Source: CAD feature listing. Evaluate the final solid. Frame: model axes, mm. Face numbers are marked on the shaded views. A direction names the side the tool comes from. Round coordinates to 2 decimals unless told otherwise and drop trailing zeros. Loops run counter-clockwise (first coordinate to the right, second up) from the corner with the lowest first, then second, coordinate; pieces in that order, holes last. Notation, with made-up numbers: (52.5, 4.5) - (109.5, 4.5) arc R16 ccw to (109.5, 21.5) - close; hole circle Ø7 at (60, 55). An arc over 180 degrees is marked (long way). Write item = value, one per line. Start each with the question number.
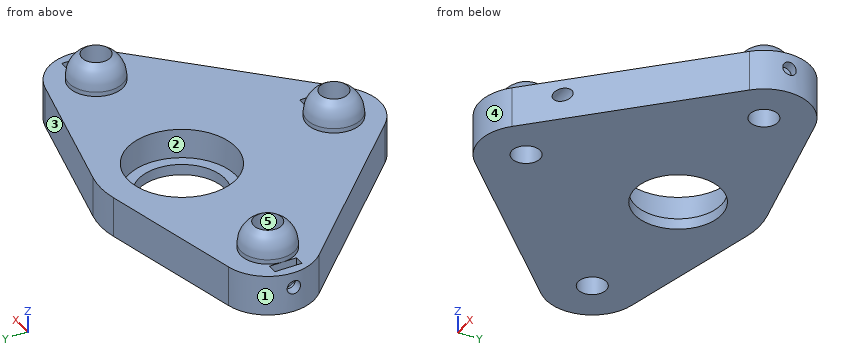
from build123d import *

# Parameters (mm, degrees)
F0_R        = 3.302
F0_R_2      = 12.7
F1_DEPTH    = 9.525
F0_R_3      = 10.16
F2_DEPTH    = 2.54
F5_DEPTH    = 8.636
F6_T1_DEPTH = 2.3368
F6_T3_DEPTH = 2.3368
F6_T5_DEPTH = 2.3368
F3_R        = 6.35
F3_R_2      = 3.302
F7_DEPTH    = 6.35
F11_R       = 1.5875
F12_DEPTH   = 6.35
F9_R        = 1.5875
F13_DEPTH   = 6.35
F10_R       = 1.5875
F14_DEPTH   = 8.382


# Not quite as in the source:
# - a fillet or chamfer that OpenCascade refuses, or shapes differently, is made with other operations: its cross-section is extruded or revolved along the edge and cut away or added
# - a feature names something its author has since deleted; it is built from what else it names


with BuildPart() as f1:
    # F0 (on Top) → F1 (new body)
    with BuildSketch(Plane.XY):
        with BuildLine():
            Line((38.3924752276, 46.5596586637), (4.3105120801, 54.476849111))
            ThreePointArc((4.3105120801, 54.476849111), (0, 54.970934), (-4.3105120801, 54.476849111))
            Line((-4.3105120801, 54.476849111), (-38.3924752276, 46.5596586637))
            ThreePointArc((-38.3924752276, 46.5596586637), (-46.4220600308, 38.9243049052), (-43.6441157783, 28.1978942818))
            Line((-43.6441157783, 28.1978942818), (-7.72300081, -7.7230397182))
            ThreePointArc((-7.72300081, -7.7230397182), (0, -10.922), (7.72300081, -7.7230397182))
            Line((7.72300081, -7.7230397182), (43.6441157783, 28.1978942818))
            ThreePointArc((43.6441157783, 28.1978942818), (46.4220600308, 38.9243049052), (38.3924752276, 46.5596586637))
        make_face()
        Circle(F0_R, mode=Mode.SUBTRACT)
        with Locations((-35.9211149683, 35.920934)):
            Circle(F0_R, mode=Mode.SUBTRACT)
        with Locations((0, 35.920934)):
            Circle(F0_R_2, mode=Mode.SUBTRACT)
        with Locations((35.9211149683, 35.920934)):
            Circle(F0_R, mode=Mode.SUBTRACT)
    extrude(amount=F1_DEPTH)

    # F0 (on Top) → F2 (join)
    with BuildSketch(Plane.XY):
        with Locations((0, 35.920934)):
            Circle(F0_R_2)
        with Locations((0, 35.920934)):
            Circle(F0_R_3, mode=Mode.SUBTRACT)
    extrude(amount=F2_DEPTH)

    # F4 (on face) → F5 (cut)
    with BuildSketch(Plane.XY.offset(9.525)):
        Polygon((-42.2711149683, 32.695134), (-42.2711149683, 35.920934), (-42.2711149683, 39.146734), (-44.6079149683, 39.146734), (-44.6079149683, 32.695134), align=None)
        Polygon((42.2711149683, 39.146734), (42.2711149683, 35.920934), (42.2711149683, 32.695134), (44.6079149683, 32.695134), (44.6079149683, 39.146734), align=None)
        Polygon((6.35, 3.2258), (6.35, 0), (6.35, -3.2258), (8.6868, -3.2258), (8.6868, 3.2258), align=None)
    extrude(amount=-F5_DEPTH, mode=Mode.SUBTRACT)

    # F6: chamfer of 3.175 x 5.499261314 on 6 edges, made by hand

    # F6_s2 → F6_t1 (join)
    with BuildSketch(Plane.YZ.offset(-44.6079149683)):
        Polygon((39.146734, 4.064), (33.647472686, 0.889), (39.146734, 0.889), align=None)
        Polygon((32.695134, 4.064), (38.194395314, 0.889), (32.695134, 0.889), align=None)
    extrude(amount=F6_T1_DEPTH)

    # F6_s4 → F6_t3 (join)
    with BuildSketch(Plane.YZ.offset(6.35)):
        Polygon((3.2258, 4.064), (-2.273461314, 0.889), (3.2258, 0.889), align=None)
        Polygon((-3.2258, 4.064), (2.273461314, 0.889), (-3.2258, 0.889), align=None)
    extrude(amount=F6_T3_DEPTH)

    # F6_s6 → F6_t5 (join)
    with BuildSketch(Plane.YZ.offset(42.2711149683)):
        Polygon((39.146734, 4.064), (33.647472686, 0.889), (39.146734, 0.889), align=None)
        Polygon((32.695134, 4.064), (38.194395314, 0.889), (32.695134, 0.889), align=None)
    extrude(amount=F6_T5_DEPTH)

    # F3 (on face) → F7 (join)
    with BuildSketch(Plane.XY.offset(9.525)):
        with Locations((-35.9211149683, 35.920934)):
            Circle(F3_R)
        with Locations((-35.9211149683, 35.920934)):
            Circle(F3_R_2, mode=Mode.SUBTRACT)
        Circle(F3_R)
        Circle(F3_R_2, mode=Mode.SUBTRACT)
        with Locations((35.9211149683, 35.920934)):
            Circle(F3_R)
        with Locations((35.9211149683, 35.920934)):
            Circle(F3_R_2, mode=Mode.SUBTRACT)
    extrude(amount=F7_DEPTH)

    # F8: fillet of radius 6.096 on 3 edges, made by hand

    # F8_s1 → F8_t2 (revolve, cut)
    with BuildSketch(Plane.XZ.offset(-35.920934)):
        with BuildLine():
            ThreePointArc((-29.5711149683, 10.5957091385), (-30.3878241069, 13.6437091385), (-32.6191149683, 15.875))
            Line((-32.6191149683, 15.875), (-29.5711149683, 15.875))
            Line((-29.5711149683, 15.875), (-29.5711149683, 10.5957091385))
        make_face()
    revolve(axis=Axis((-35.9211149683, 35.920934, 15.875), (0, 0, 1)), mode=Mode.SUBTRACT)

    # F8_s3 → F8_t4 (revolve, cut)
    with BuildSketch(Plane.XZ.offset(-35.920934)):
        with BuildLine():
            ThreePointArc((42.2711149683, 10.5957091385), (41.4544058298, 13.6437091385), (39.2231149683, 15.875))
            Line((39.2231149683, 15.875), (42.2711149683, 15.875))
            Line((42.2711149683, 15.875), (42.2711149683, 10.5957091385))
        make_face()
    revolve(axis=Axis((35.9211149683, 35.920934, 15.875), (0, 0, 1)), mode=Mode.SUBTRACT)

    # F8_s5 → F8_t6 (revolve, cut)
    with BuildSketch(Plane.XZ):
        with BuildLine():
            ThreePointArc((6.35, 10.5957091385), (5.5332908615, 13.6437091385), (3.302, 15.875))
            Line((3.302, 15.875), (6.35, 15.875))
            Line((6.35, 15.875), (6.35, 10.5957091385))
        make_face()
    revolve(axis=Axis((0, 0, 15.875), (0, 0, 1)), mode=Mode.SUBTRACT)

    # F11 (on face) → F12 (cut, symmetric)
    with BuildSketch(Plane(origin=(44.6079149683, 0, 0), x_dir=(0, -1, 0), z_dir=(-1, 0, 0))):
        with Locations((-35.8627085169, 5.8928)):
            Circle(F11_R)
    extrude(amount=F12_DEPTH, both=True, mode=Mode.SUBTRACT)

    # F9 (on face) → F13 (cut, symmetric)
    with BuildSketch(Plane.YZ.offset(-44.6079149683)):
        with Locations((35.8627085169, 5.8928)):
            Circle(F9_R)
    extrude(amount=F13_DEPTH, both=True, mode=Mode.SUBTRACT)

    # F10 (on face) → F14 (cut, symmetric)
    with BuildSketch(Plane(origin=(8.6868, 0, 0), x_dir=(0, -1, 0), z_dir=(-1, 0, 0))):
        with Locations((0.0582254831, 5.8928)):
            Circle(F10_R)
    extrude(amount=F14_DEPTH, both=True, mode=Mode.SUBTRACT)


solid = f1.part
(1) Material intervals for line 1 along Y through (x, z) = (-1.5, 1); line 2 along Y through (x, z) = (-2.5, 6); line 3 along X through (y, z) = (34.5, 12.5), sorted ascending. Write a range as from..to.
(2) Mould query, pull axis X, two halves, no side actions, for the marked faces 3, 4 and 5. Classes: +X half, -X half, draft (parallel to the pull), parting line (faces both ways), or undercut.
(3) Cut plane D-D (x = 16). Output: boundary loops of the cut face in (y, z) (1 decimal), and give its area (3 significant figures).
(4) Cut plane A-A (z = 8.5). Output: boundary loops of the cut face in (x, y), and give its area (3 significant figures).
(5) Access query for the marked faces 1 and 2. Directions: +Z, -Z, +X, -X, +Y, -Y. A direction counts if a zero-diameter tool reaches every point of the face in a straight line with its end or side. Return the directions, or none.
(6) Cut plane C-C (y = 15.5). Output: boundary loops of the cut face in (x, z) (3 decimals), and give its area (3 significant figures).
(7) Cut plane B-B (x = 0). State how many separate pieces and enclosed holes the cut face has, and give its area (3 significant figures).
(8) Pin query (flat end, axial travel): P1, Ø10, axis at x = -17, y = 14, coming from the +Z side (3 decimals); P2, Ø3, axis at y = 35.86, z = 5.89, coming from the +X side; P3, Ø3, axis at y = 35.86, z = 5.89, coming from the -X side; P4, Ø15, axis at x = 0, y = 35.92, coming from the +Z side. Return the tip coordinate at first contact, or that it passes through.
Solution:
q1.line_1 = -10.82..-2.94, 2.94..25.87, 45.97..54.91
q1.line_2 = -10.63..-2.16, 2.16..23.47, 48.37..54.81
q1.line_3 = -41.8..-38.9, -32.94..-30.05, 30.05..32.94, 38.9..41.8
q2.face_3 = +X half
q2.face_4 = parting line
q2.face_5 = undercut
q3.outline = (0.6, 0) - (51.8, 0) - (51.8, 9.5) - (0.6, 9.5) - (0.6, 7.4) arc R1.6 cw to (0.6, 4.4) - close
q3.area = 486 mm^2
q4.outline = (-43.64, 28.2) - (-7.72, -7.72) arc R10.92 ccw to (7.72, -7.72) - (43.64, 28.2) arc R10.92 ccw to (38.39, 46.56) - (4.31, 54.48) arc R19.05 ccw to (-4.31, 54.48) - (-38.39, 46.56) arc R10.92 ccw to start; hole (-44.61, 32.7) - (-42.27, 32.7) - (-42.27, 39.15) - (-44.61, 39.15) - close; hole circle Ø6.6 at (-35.92, 35.92); hole circle Ø25.4 at (0, 35.92); hole circle Ø6.6 at (0, 0); hole (6.35, -3.23) - (8.69, -3.23) - (8.69, 3.23) - (6.35, 3.23) - close; hole circle Ø6.6 at (35.92, 35.92); hole (42.27, 32.7) - (44.61, 32.7) - (44.61, 39.15) - (42.27, 39.15) - close
q4.area = 3,220 mm^2
q5.face_1 = +Z, -Z, -X
q5.face_2 = +Z
q6.outline = (-30.946, 0) - (30.946, 0) - (30.946, 9.525) - (-30.946, 9.525) - close
q6.area = 590 mm^2
q7.separate_pieces = 3
q7.enclosed_holes = 0
q7.area = 365 mm^2
q8.P1 = 9.525
q8.P2 = 33.01
q8.P3 = -33.01
q8.P4 = through
